CAD build for the part. Positions are in the model's coordinates, mm. A direction names the side the tool comes from. Give positions to 0.01 mm unless a question says otherwise; leave off trailing zeros. Loops run counter-clockwise (first coordinate to the right, second up) from the corner with the lowest first, then second, coordinate; pieces in that order, holes last.
```python
from build123d import *

# Parameters (mm, degrees)
BOSS_EXTRUDE1_DEPTH = 6.35
SKETCH3_R           = 1.27
CUT_EXTRUDE2_DEPTH  = 6.35


with BuildPart() as part:
    # Sketch1 → Boss-Extrude1 (new body)
    with BuildSketch(Plane(origin=(0, 0, 0), x_dir=(1, 0, 0), z_dir=(0, 1, 0))):
        Polygon((0, 0), (-57.15, 0), (-57.15, 49.53), (-50.8, 49.53), (-50.8, 6.35), (0, 6.35), align=None)
    extrude(amount=BOSS_EXTRUDE1_DEPTH)

    # Sketch3 → Cut-Extrude2 (cut)
    with BuildSketch(Plane.ZY.offset(57.15)):
        with Locations((-42.926, 3.072725117)):
            Circle(SKETCH3_R)
        with Locations((-11.938, 3.072725117)):
            Circle(SKETCH3_R)
    extrude(amount=-CUT_EXTRUDE2_DEPTH, mode=Mode.SUBTRACT)


solid = part.part
```
1. Pull direction Z, two halves, no side cores. Call faces 1 (the face through (-41, 0, -5)), 2 (the face through (-54, 3, -49.53)), 3 (the face through (-54.019, 3.129, -44.195)): released by +Z, released by -Z, zero draft, split by the parting line, or undercut.
Responses:
face 1: zero draft
face 2: released by -Z
face 3: undercut
2. Saw through at B-B, the plane x = -10.5. List the corners of the cut face in (y, z).
Responses:
outline: (0, -6.35) - (6.35, -6.35) - (6.35, 0) - (0, 0) - close
3. Drop a flat-ended pin along its axis: pin 1 (1.9 mm diameter, centred on x = -22.5, y = 2, fed in from -Z). Give the stop position or say it passes through.
Responses:
pin 1: stops at z = -6.35
4. Saw through at C-C, the plane z = -21.5. List the corners of the cut face in (x, y), and give its area (3 significant figures).
Responses:
outline: (-57.15, 0) - (-50.8, 0) - (-50.8, 6.35) - (-57.15, 6.35) - close
area: 40.3 mm2
5. Tool access for faces 4 (the face through (-50.8, 3, -28)), 5 (the face through (-28, 3, 0)): list every direction of +Z, -Z, +X, -X, +Y, -Y with a clear straight run to the whole face (end or side of a thin tool).
Responses:
face 4: -Z, +X, +Y, -Y
face 5: +Z, +X, -X, +Y, -Y
6. Saw through at A-A, the plane y = 5. List the corners of the cut face in (x, z).
Responses:
outline: (-57.15, -49.53) - (-50.8, -49.53) - (-50.8, -6.35) - (0, -6.35) - (0, 0) - (-57.15, 0) - close
7. Probe line 1 along Z through (x, y) = (-13, 4.5); line 2 along X through (y, z) = (1.75, -8). List the from-to ranges inside material, lowest first.
Responses:
line 1: z = -6.35 to 0
line 2: x = -57.15 to -50.8
